from build123d import *

# Parameters (mm, degrees)
SKETCH1_R           = 8
BOSS_EXTRUDE1_DEPTH = 105
SKETCH2_R           = 12.5
BOSS_EXTRUDE2_DEPTH = 8
CHAMFER1_SIZE       = 1
SKETCH3_R           = 2
CUT_EXTRUDE1_DEPTH  = 500


with BuildPart() as part:
    # Sketch1 → Boss-Extrude1 (new body)
    with BuildSketch(Plane.XY):
        Circle(SKETCH1_R)
    extrude(amount=BOSS_EXTRUDE1_DEPTH)

    # Sketch2 → Boss-Extrude2 (add)
    with BuildSketch(Plane.XY.offset(105)):
        Circle(SKETCH2_R)
    extrude(amount=BOSS_EXTRUDE2_DEPTH)

    # Chamfer1
    chamfer1_edges = [part.edges().sort_by_distance(p)[0] for p in [
        (-12.5, 0, 113),
    ]]
    chamfer(chamfer1_edges, length=CHAMFER1_SIZE)

    # Sketch3 → Cut-Extrude1 (cut, symmetric)
    with BuildSketch(Plane(origin=(0, 0, 0), x_dir=(0, 0, -1), z_dir=(1, 0, 0))):
        with Locations(Location((-11, 0, 0), (0, 0, 180))):
            Circle(SKETCH3_R)
    extrude(amount=CUT_EXTRUDE1_DEPTH, both=True, mode=Mode.SUBTRACT)


solid = part.part
CAD build for the part. Positions are in the model's coordinates, mm. A direction names the side the tool comes from. Coordinates: 2 decimals unless noted, no trailing zeros. Order: outer loops, then holes, each group sorted by start corner. A loop starts at its lowest first (then second) coordinate and runs counter-clockwise, first axis right, second up. Notation, with made-up numbers: (21, -14.5) -> (69, -14.5) arc R22 ccw to (69, 11.5) -> close; hole circle Ø2 at (47.25, 17). An arc over 180 degrees is marked (long way). Answer in a Markdown table with one row per item.
1) Drill centre lines: line 1 (Y direction, x = 1, z = 11); line 2 (X direction, y = 0.25, z = 33.5); line 3 (Y direction, x = -4.5, z = 11). Where is each one in solid material? Low to high.
Check values:
| item | result |
|---|---|
| line 1 | -7.94 to -2, 2 to 7.94 |
| line 2 | -8 to 8 |
| line 3 | -6.61 to -2, 2 to 6.61 |
2) Mould opens along Z. For faces 1 (the face through (-0.2, -8.2, 105)), 2 (the face through (0, 0, 113)), 3 (the face through (0.1, 1.2, 9.4)) say: pulls with the +Z half, pulls with the -Z half, needs draft (parallel to the pull), parting line crosses it, or undercut.
Check values:
| item | result |
|---|---|
| face 1 | pulls with the -Z half |
| face 2 | pulls with the +Z half |
| face 3 | undercut |
3) Band-saw the part on D-D (z = 11). List the corners of the cut face in (x, y), and give its area (3 significant figures).
Check values:
| item | result |
|---|---|
| outline | (-7.75, -2) arc R8 ccw to (7.75, -2) -> close; (-7.75, 2) -> (7.75, 2) arc R8 ccw to start |
| area | 138 mm2 |
4) Band-saw the part on C-C (z = 64). List the corners of the cut face in (x, y).
Check values:
| item | result |
|---|---|
| outline | circle Ø16 at (0, 0) |
5) Band-saw the part on B-B (x = 0). List the corners of the cut face in (y, z), and give its area (3 significant figures).
Check values:
| item | result |
|---|---|
| outline | (-12.5, 105) -> (-8, 105) -> (-8, 0) -> (8, 0) -> (8, 105) -> (12.5, 105) -> (12.5, 112) -> (11.5, 113) -> (-11.5, 113) -> (-12.5, 112) -> close; hole circle Ø4 at (0, 11) |
| area | 1,870 mm2 |
6) Band-saw the part on A-A (y = 0). List the corners of the cut face in (x, z), and give its area (4 significant figures).
Check values:
| item | result |
|---|---|
| outline | (-12.5, 105) -> (-8, 105) -> (-8, 13) -> (8, 13) -> (8, 105) -> (12.5, 105) -> (12.5, 112) -> (11.5, 113) -> (-11.5, 113) -> (-12.5, 112) -> close; (-8, 0) -> (8, 0) -> (8, 9) -> (-8, 9) -> close |
| area | 1,815 mm2 |
7) Flat gauge pins, fed straight in: P1, Ø5, axis at x = 3.5, z = 76.5, coming from the +Y side; P2, Ø6.5, axis at y = 0, z = 11, coming from the -X side; P3, Ø4, axis at x = -2, z = 80.5, coming from the +Y side. Where does each tip first touch, or does it go through?
Check values:
| item | result |
|---|---|
| P1 | y = 7.94 |
| P2 | x = -8 |
| P3 | y = 8 |
8) Which spindle directions (+Z, -Z, +X, -X, +Y, -Y) get a long thin tool onto all of the face, cutting with end or side? Do faces 4 (the face through (-1.73, -7.81, 51.76)), 5 (the face through (0, 0, 0)). Say none if no direction does.
Check values:
| item | result |
|---|---|
| face 4 | -Z |
| face 5 | -Z, +X, -X, +Y, -Y |
